Source: three-view drawing plus pictorial views. Frame: mm from the lowest corner of the part. A direction names the side the tool comes from. Give positions to 0.01 mm unless a question says otherwise; leave off trailing zeros. Order: outer loops, then holes, each group sorted by start corner. A loop starts at its lowest first (then second) coordinate and runs counter-clockwise, first axis right, second up. Notation, with made-up numbers: M 28,19 L 77,19 A23 cw 77,29 Z; hole C 47,0 d10. An arc over 180 degrees is marked long. Use CSV: the item, a comma, the result in double quotes. Start each with the question number.
1. Section query A-A, the plane x = 12.5. Return the cut outline in (y, z).
2. Reachability of the marked faces 1 and 2 from +Z, -Z, +X, -X, +Y, -Y: full face, straight path, thin tool, end or side. Return the list, or none.
3. Section query B-B, the plane z = 22. Return the cut outline in (x, y), plus the area to 3 significant figures.
4. Line query: line 1 along Y through (x, z) = (1.5, 22); line 2 along X through (y, z) = (55.75, 32); line 3 along X through (y, z) = (17, 56.5). Output: solid intervals per line, ascending. Write a range as [from, to].
5. Section query D-D, the plane y = 53. Return the cut outline in (x, z).
6. Pin query (flat end, axial travel): P1, Ø8, axis at x = 4.5, z = 42.5, coming from the +Y side; P2, Ø7, axis at y = 19.5, z = 50, coming from the +X side; P3, Ø4.5, axis at x = 4.5, y = 60, coming from the -Z side. Return the tip coordinate at first contact, or that it passes through.
7. Mould query, pull axis Y, two halves, no side actions, for the marked faces 3, 4 and 5. Classes: released by +Y, released by -Y, zero draft, split by the parting line, or undercut.
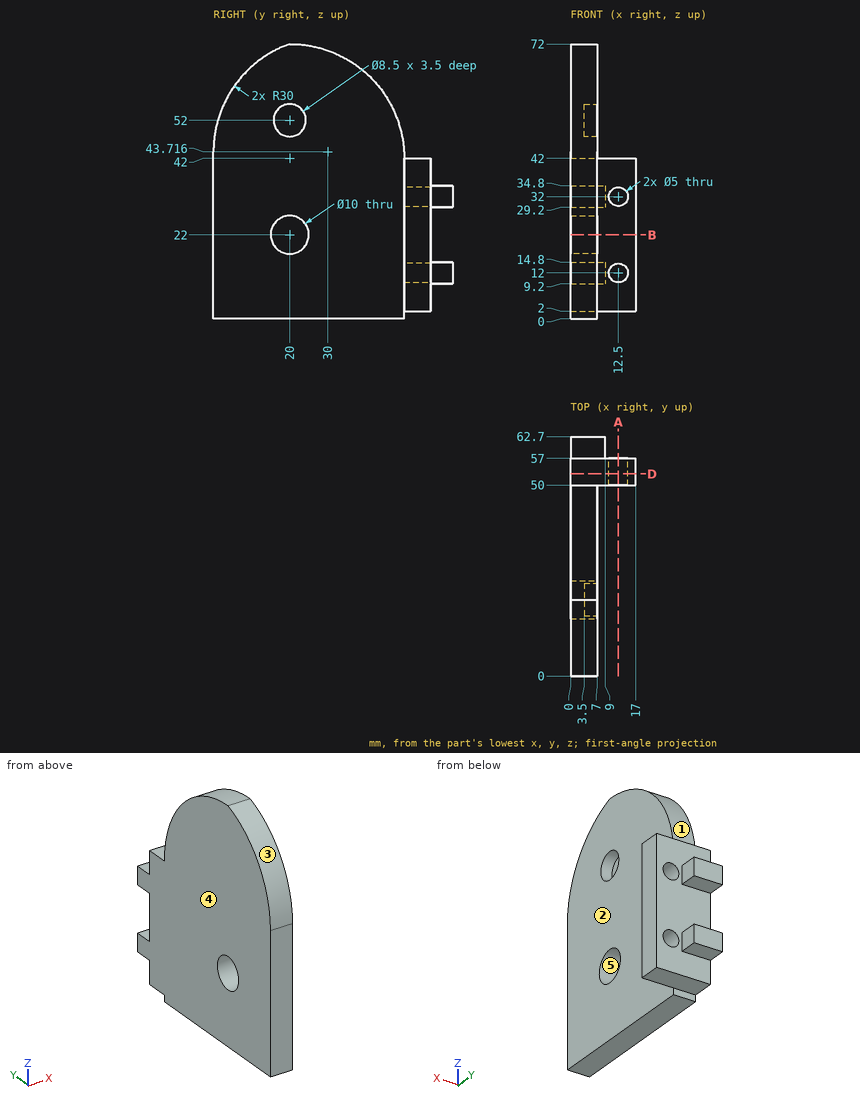
Result set:
1,outline,"M 50,2 L 57,2 L 57,9.5 L 50,9.5 Z; M 50,14.5 L 57,14.5 L 57,29.5 L 50,29.5 Z; M 50,34.5 L 57,34.5 L 57,42 L 50,42 Z"
2,face 1,"+Z, +X, -X, +Y"
2,face 2,"+Z, -Z, +X, -Y"
3,outline,"M 0,0 L 7,0 L 7,15 L 0,15 Z; M 0,25 L 7,25 L 7,50 L 17,50 L 17,57 L 0,57 Z"
3,area,"399 mm2"
4,line 1,"[0, 15], [25, 57]"
4,line 2,"[0, 10], [15, 17]"
4,line 3,"[0, 7]"
5,outline,"M 0,2 L 17,2 L 17,42 L 0,42 Z; hole C 12.5,12 d5; hole C 12.5,32 d5"
6,P1,"y = 57"
6,P2,"x = 7"
6,P3,"z = 9.2"
7,face 3,"released by -Y"
7,face 4,"zero draft"
7,face 5,"undercut"
